from build123d import *

# Parameters (mm, degrees)
SKETCH1_W           = 36.8
SKETCH1_H           = 39.7
BOSS_EXTRUDE1_DEPTH = 4.8
SKETCH2_W           = 44.7
SKETCH2_H           = 3.9
BOSS_EXTRUDE2_DEPTH = 20
CUT_EXTRUDE1_REACH  = 58.226
CHAMFER1_SIZE       = 2.85
CUT_EXTRUDE2_DEPTH  = 58.709011428
FILLET1_R           = 2


with BuildPart() as part:
    # Sketch1 → Boss-Extrude1 (new body)
    with BuildSketch(Plane(origin=(0, 0, 0), x_dir=(1, 0, 0), z_dir=(0, 1, 0))):
        with Locations((18.4, 19.85)):
            Rectangle(SKETCH1_W, SKETCH1_H)
    extrude(amount=BOSS_EXTRUDE1_DEPTH)

    # Sketch2 → Boss-Extrude2 (add)
    with BuildSketch(Plane(origin=(0, 0, 0), x_dir=(1, 0, 0), z_dir=(0, 1, 0))):
        with Locations((14.45, 37.75)):
            Rectangle(SKETCH2_W, SKETCH2_H)
        with Locations((14.45, 1.95)):
            Rectangle(SKETCH2_W, SKETCH2_H)
    extrude(amount=BOSS_EXTRUDE2_DEPTH)

    # Sketch3 → Cut-Extrude1 (cut, up to next)
    with BuildSketch(Plane(origin=(0, 4.8, 0), x_dir=(1, 0, 0), z_dir=(0, 1, 0)), mode=Mode.PRIVATE) as cut_extrude1_sk1:
        with BuildLine():
            Line((26.45, 14.5), (29.05, 14.5))
            ThreePointArc((29.05, 14.5), (31.8, 11.75), (29.05, 9))
            Line((29.05, 9), (26.45, 9))
            ThreePointArc((26.45, 9), (23.7, 11.75), (26.45, 14.5))
        make_face()
    cut_extrude1_tool1 = extrude(cut_extrude1_sk1.sketch, amount=-CUT_EXTRUDE1_REACH, mode=Mode.PRIVATE) & part.part
    # Sketch3 → Cut-Extrude1 (cut, up to next)
    with BuildSketch(Plane(origin=(0, 4.8, 0), x_dir=(1, 0, 0), z_dir=(0, 1, 0)), mode=Mode.PRIVATE) as cut_extrude1_sk2:
        with BuildLine():
            Line((18.7, 29.35), (18.7, 26.75))
            ThreePointArc((18.7, 26.75), (15.95, 24), (13.2, 26.75))
            Line((13.2, 26.75), (13.2, 29.35))
            ThreePointArc((13.2, 29.35), (15.95, 32.1), (18.7, 29.35))
        make_face()
    cut_extrude1_tool2 = extrude(cut_extrude1_sk2.sketch, amount=-CUT_EXTRUDE1_REACH, mode=Mode.PRIVATE) & part.part
    add(cut_extrude1_tool1.solids().sort_by_distance((27.75, 4.8, -11.75))[0], mode=Mode.SUBTRACT)
    add(cut_extrude1_tool2.solids().sort_by_distance((15.95, 4.8, -28.05))[0], mode=Mode.SUBTRACT)

    # Chamfer1
    chamfer1_edges = [part.edges().sort_by_distance(p)[0] for p in [
        (23.7, 4.8, -11.75),
        (27.75, 4.8, -9),
        (31.8, 4.8, -11.75),
        (27.75, 4.8, -14.5),
        (15.95, 4.8, -32.1),
        (13.2, 4.8, -28.05),
        (15.95, 4.8, -24),
        (18.7, 4.8, -28.05),
    ]]
    chamfer(chamfer1_edges, length=CHAMFER1_SIZE)

    # Sketch4 → Cut-Extrude2 (cut, through all)
    with BuildSketch(Plane(origin=(0, 0, -39.7), x_dir=(-1, 0, 0), z_dir=(0, 0, -1))):
        Polygon((-36.8, 20), (-36.8, 7.5), (-15.8, 20), align=None)
    extrude(amount=-CUT_EXTRUDE2_DEPTH, mode=Mode.SUBTRACT)

    # Fillet1
    fillet1_edges = [part.edges().sort_by_distance(p)[0] for p in [
        (15.8, 20, -37.75),
        (15.8, 20, -1.95),
        (36.8, 7.5, -37.75),
        (36.8, 7.5, -1.95),
    ]]
    fillet(fillet1_edges, radius=FILLET1_R)


solid = part.part
CAD build for the part. Positions are in the model's coordinates, mm. A direction names the side the tool comes from. Coordinates: 2 decimals unless noted, no trailing zeros. Order: outer loops, then holes, each group sorted by start corner. A loop starts at its lowest first (then second) coordinate and runs counter-clockwise, first axis right, second up. Notation, with made-up numbers: (39, 59.5) -> (92, 59.5) arc R26 cw to (92, 93.5) -> close; hole circle Ø3 at (-40, -8). An arc over 180 degrees is marked (long way). Answer in a Markdown table with one row per item.
1) Which spindle directions (+Z, -Z, +X, -X, +Y, -Y) get a long thin tool onto all of the face, cutting with end or side? Do faces 1 (the face through (16.03, 2.72, -23.23)), 2 (the face through (31.8, 1, -11.8)), 3 (the face through (0, 2, -20)), 4 (the face through (36.546, 7.339, -1.923)), 5 (the face through (18, 4.8, -20)). Say none if no direction does.
Check values:
| item | result |
|---|---|
| face 1 | +Y |
| face 2 | +Y, -Y |
| face 3 | -X, +Y, -Y |
| face 4 | +Z, -Z, +X, +Y |
| face 5 | +X, -X, +Y |
2) Mould opens along Z. For faces 6 (the face through (14, 10, -39.7)), 7 (the face through (-7.9, 10, -38)), 8 (the face through (27.77, 3.36, -7.59)) say: pulls with the +Z half, pulls with the -Z half, needs draft (parallel to the pull), parting line crosses it, or undercut.
Check values:
| item | result |
|---|---|
| face 6 | pulls with the -Z half |
| face 7 | needs draft |
| face 8 | undercut |
3) Flat gauge pins, fed straight in: P1, Ø5.5, axis at y = 2, z = -25, coming from the -X side; P2, Ø9.5, axis at x = 13, z = -24, coming from the +Y side. Where does each tip first touch, or does it go through?
Check values:
| item | result |
|---|---|
| P1 | x = 0 |
| P2 | y = 4.8 |
4) Drill centre lines: line 1 (Z direction, x = -4, y = 14.75); line 2 (Y direction, x = 4, z = -11); line 3 (Z direction, x = 26, y = 2.75). Where is each one in solid material? Low to high.
Check values:
| item | result |
|---|---|
| line 1 | -39.7 to -35.8, -3.9 to 0 |
| line 2 | 0 to 4.8 |
| line 3 | -39.7 to -15.27, -8.23 to 0 |
5) Band-saw the part on C-C (z = -11.75). List the corners of the cut face in (x, y).
Check values:
| item | result |
|---|---|
| outline | (0, 0) -> (23.7, 0) -> (23.7, 1.95) -> (20.85, 4.8) -> (0, 4.8) -> close; (31.8, 0) -> (36.8, 0) -> (36.8, 4.8) -> (34.65, 4.8) -> (31.8, 1.95) -> close |
6) Band-saw the part on B-B (y = 9). List the corners of the cut face in (x, z).
Check values:
| item | result |
|---|---|
| outline | (-7.9, -39.7) -> (34.28, -39.7) -> (34.28, -35.8) -> (-7.9, -35.8) -> close; (-7.9, -3.9) -> (34.28, -3.9) -> (34.28, 0) -> (-7.9, 0) -> close |
7) Band-saw the part on A-A (x = -4). List the corners of the cut face in (y, z).
Check values:
| item | result |
|---|---|
| outline | (0, -39.7) -> (20, -39.7) -> (20, -35.8) -> (0, -35.8) -> close; (0, -3.9) -> (20, -3.9) -> (20, 0) -> (0, 0) -> close |
